```python
from build123d import *

# Parameters (mm, degrees)
ESQUISSE8_R        = 1.5
ESQUISSE8_W        = 8
ESQUISSE8_H        = 3
ESQUISSE8_W_2      = 5
BOSS_EXTRU_8_DEPTH = 3


with BuildPart() as part:
    # Esquisse8 → Boss.-Extru.8 (new body)
    with BuildSketch(Plane.XY):
        with BuildLine():
            Line((-62.973836854, -34.551748671), (17.026163146, -34.551748671))
            ThreePointArc((17.026163146, -34.551748671), (23.026163146, -40.551748671), (17.026163146, -46.551748671))
            Line((17.026163146, -46.551748671), (-62.973836854, -46.551748671))
            ThreePointArc((-62.973836854, -46.551748671), (-68.973836854, -40.551748671), (-62.973836854, -34.551748671))
        make_face()
        with Locations((-62.973836854, -40.551748671)):
            Circle(ESQUISSE8_R, mode=Mode.SUBTRACT)
        with Locations((-30.973836854, -40.457603156)):
            Circle(ESQUISSE8_R, mode=Mode.SUBTRACT)
        with Locations((17.026163146, -40.551748671)):
            Circle(ESQUISSE8_R, mode=Mode.SUBTRACT)
        with Locations((-48.973836854, -40.551748671)):
            Rectangle(ESQUISSE8_W, ESQUISSE8_H, mode=Mode.SUBTRACT)
        with Locations((4.526163146, -40.551748671)):
            Rectangle(ESQUISSE8_W_2, ESQUISSE8_H, mode=Mode.SUBTRACT)
    extrude(amount=BOSS_EXTRU_8_DEPTH)


solid = part.part
```
Part model, mm, in its own coordinate system. A direction names the side the tool comes from. Give positions to 0.01 mm unless a question says otherwise; leave off trailing zeros. Order: outer loops, then holes, each group sorted by start corner. A loop starts at its lowest first (then second) coordinate and runs counter-clockwise, first axis right, second up. Notation, with made-up numbers: M 89,-27 L 124,-27 A17 cw 124,-12 Z; hole C 67.5,-12.5 d7. An arc over 180 degrees is marked long. Use a Markdown table: item, result. Add a question column.
(1) 3-axis set-ups, long thin cutter, end or side, ignore diameter. For faces 5 (the face through (23, -40, 1)), 6 (the face through (-49, -39.052, 1)): which of +Z, -Z, +X, -X, +Y, -Y reach the whole face in a straight line?
(2) Saw through at D-D, the plane y = -44. Give the cut face in (x, z).
(3) Probe line 1 along X through (y, z) = (-40.5, 2.45); line 2 along Y through (x, z) = (-63, 1.55); line 3 along X through (y, z) = (-39.5, 1.85). List the from-to ranges inside material, lowest first. Write a range as [from, to].
(4) Saw through at C-C, the plane y = -36. Give the cut face in (x, z), and give its area (3 significant figures).
(5) Mould opens along Y. For faces 1 (the face through (-22, -40, 0)), 2 (the face through (-52.974, -41, 1)), 3 (the face through (-68.972, -40.684, 1.479)), 4 (the face through (-22, -46.552, 1)) say: +Y half, -Y half, draft (parallel to the pull), parting line (faces both ways), or undercut.
(6) Saw through at B-B, the plane z = 1.95. Give the cut face in (x, y), and give its area (3 significant figures).
(7) Saw through at A-A, the plane x = -46. Give the cut face in (y, z).
Answer key:
| question | item | result |
|---|---|---|
| 1 | face 5 | +Z, -Z, +X |
| 1 | face 6 | +Z, -Z |
| 2 | outline | M -67.88,0 L 21.94,0 L 21.94,3 L -67.88,3 Z |
| 3 | line 1 | [-68.97, -64.47], [-61.47, -52.97], [-44.97, -32.47], [-29.47, 2.03], [7.03, 15.53], [18.53, 23.03] |
| 3 | line 2 | [-46.55, -42.05], [-39.05, -34.55] |
| 3 | line 3 | [-68.88, -64.04], [-61.9, -52.97], [-44.97, -32.13], [-29.82, 2.03], [7.03, 15.96], [18.1, 22.93] |
| 4 | outline | M -66.88,0 L 20.94,0 L 20.94,3 L -66.88,3 Z |
| 4 | area | 263 mm^2 |
| 5 | face 1 | draft |
| 5 | face 2 | undercut |
| 5 | face 3 | parting line |
| 5 | face 4 | -Y half |
| 6 | outline | M -62.97,-46.55 L 17.03,-46.55 A6 ccw 17.03,-34.55 L -62.97,-34.55 A6 ccw Z; hole C -62.97,-40.55 d3; hole M -52.97,-42.05 L -44.97,-42.05 L -44.97,-39.05 L -52.97,-39.05 Z; hole C -30.97,-40.46 d3; hole M 2.03,-42.05 L 7.03,-42.05 L 7.03,-39.05 L 2.03,-39.05 Z; hole C 17.03,-40.55 d3 |
| 6 | area | 1,010 mm^2 |
| 7 | outline | M -46.55,0 L -42.05,0 L -42.05,3 L -46.55,3 Z; M -39.05,0 L -34.55,0 L -34.55,3 L -39.05,3 Z |
